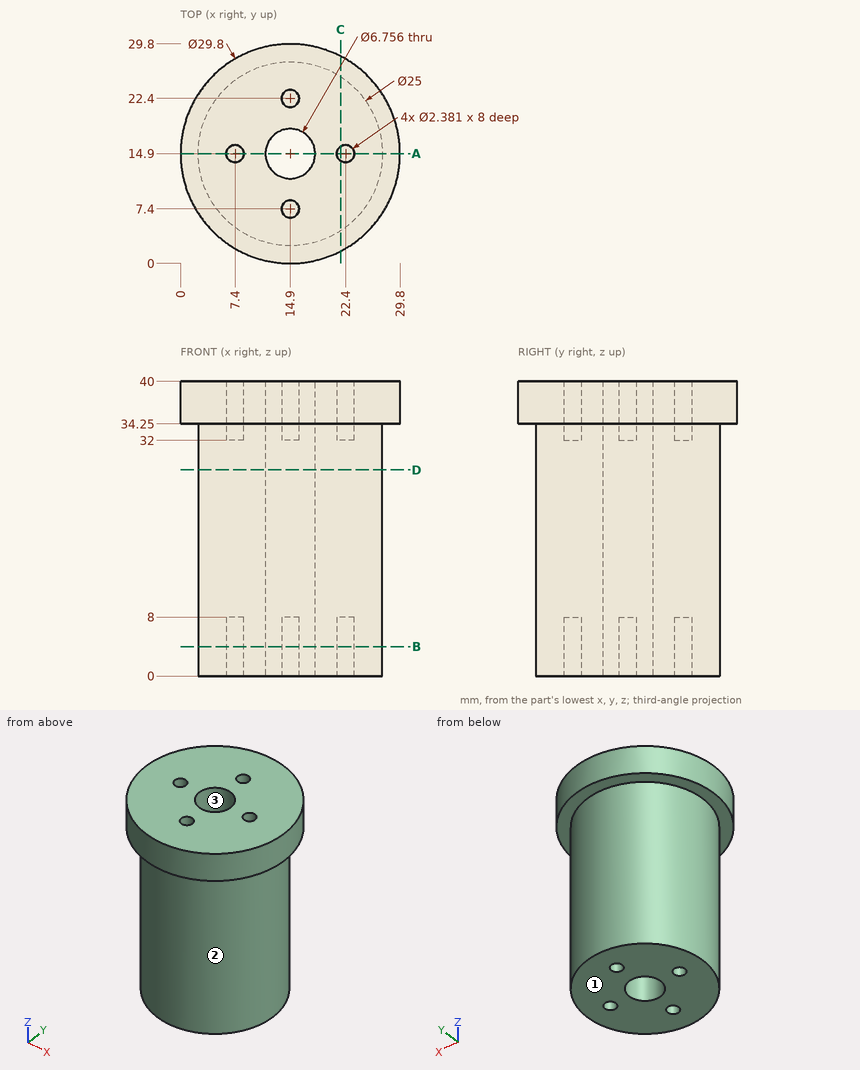
Could you check a few things on this drawing? It's one solid part, dimensions in mm from its lowest x, y, z. Give positions to 0.01 mm unless a question says otherwise; leave off trailing zeros. Loops run counter-clockwise (first coordinate to the right, second up) from the corner with the lowest first, then second, coordinate; pieces in that order, holes last. Notation, with made-up numbers: M -6.75,82.25 L 38.25,82.25 A10 ccw 38.25,98.25 Z; hole C 16,79.25 d2. An arc over 180 degrees is marked long. Return JSON: item names as keys, results as strings.
Item 1: Thinking about a two-plate mould opening in Y: for the marked faces 1, 2 and 3, which applies, released by +Y, released by -Y, zero draft, split by the parting line, or undercut?
A:
{"face 1": "zero draft", "face 2": "split by the parting line", "face 3": "undercut"}
Item 2: Imagine slicing it at B-B on z = 4. List the corners of the cut face in (x, y) for me.
A:
{"outline": "C 14.9,14.9 d25; hole C 7.4,14.9 d2.38; hole C 14.9,14.9 d6.76; hole C 14.9,7.4 d2.38; hole C 14.9,22.4 d2.38; hole C 22.4,14.9 d2.38"}
Item 3: Imagine slicing it at C-C on x = 21.75. List the corners of the cut face in (y, z) for me.
A:
{"outline": "M 1.67,34.25 L 4.44,34.25 L 4.44,0 L 13.9,0 L 13.9,8 L 15.9,8 L 15.9,0 L 25.36,0 L 25.36,34.25 L 28.13,34.25 L 28.13,40 L 15.9,40 L 15.9,32 L 13.9,32 L 13.9,40 L 1.67,40 Z"}
Item 4: Please list where these lines run through material, in increasing order: line 1 (X direction, y = 7.4, z = 35.75) (1 decimal); line 2 (X direction, y = 12, z = 12) (1 decimal); line 3 (Y direction, x = 22.4, z = 2.75).
A:
{"line 1": "x = 2 to 13.7, 16.1 to 27.8", "line 2": "x = 2.7 to 13.2, 16.6 to 27.1", "line 3": "y = 4.9 to 13.71, 16.09 to 24.9"}
Item 5: Imagine slicing it at D-D on z = 28. List the corners of the cut face in (x, y) for me, then the cut area to 3 significant figures.
A:
{"outline": "C 14.9,14.9 d25; hole C 14.9,14.9 d6.76", "area": "455 mm^2"}
Item 6: I'm going to push flat-ended pins straight in: pin 1 Ø1.9 at (x, y) = (22.4, 14.9) entering from -Z; pin 2 Ø1.5 at (x, z) = (4, 35) entering from -Y; pin 3 Ø1.5 at (y, z) = (15, 17) entering from -X; pin 4 Ø5.5 at (x, y) = (14.9, 14.9) entering from -Z. Where does each tip first touch, or does it pass through?
A:
{"pin 1": "stops at z = 8", "pin 2": "stops at y = 3.99", "pin 3": "stops at x = 2.4", "pin 4": "passes through"}
Item 7: Imagine slicing it at A-A on y = 14.9. List the corners of the cut face in (x, z) for me.
A:
{"outline": "M 0,34.25 L 2.4,34.25 L 2.4,0 L 6.21,0 L 6.21,8 L 8.59,8 L 8.59,0 L 11.52,0 L 11.52,40 L 8.59,40 L 8.59,32 L 6.21,32 L 6.21,40 L 0,40 Z; M 18.28,0 L 21.21,0 L 21.21,8 L 23.59,8 L 23.59,0 L 27.4,0 L 27.4,34.25 L 29.8,34.25 L 29.8,40 L 23.59,40 L 23.59,32 L 21.21,32 L 21.21,40 L 18.28,40 Z"}
